```python
from build123d import *

# Parameters (mm, degrees)
SWEEP_THIN1_PROFILE_R   = 30
SWEEP_THIN1_PROFILE_R_2 = 29


with BuildPart() as part:
    # Sweep-Thin1: sweep along a curve in space
    with BuildLine() as sweep_thin1_path:
        Line((-30068.540907505, -16257.859563295, 40521.703196056), (-29659.188972505, -16257.859563295, 40521.703196056))
        ThreePointArc((-29599.188972505, -16197.859563295, 40521.703196056), (-29616.762565634, -16240.285970167, 40521.703196056), (-29659.188972505, -16257.859563295, 40521.703196056))
        Line((-29599.188972505, -16197.859563295, 40521.703196056), (-29599.188972505, -16134.686242211, 40521.703196056))
    # Sweep-Thin1 profile (on start of the path) → Sweep-Thin1 (sweep)
    with BuildSketch(Plane(origin=(-30068.540907505, -16257.859563295, 40521.703196056), x_dir=(0, 0, 1), z_dir=(1, 0, 0))):
        Circle(SWEEP_THIN1_PROFILE_R)
        Circle(SWEEP_THIN1_PROFILE_R_2, mode=Mode.SUBTRACT)
    sweep(path=sweep_thin1_path.line)


solid = part.part
```
Check sheet for the modelled part. Datum: model origin and axes. Units: mm. A direction names the side the tool comes from. Give positions to 0.01 mm unless a question says otherwise; leave off trailing zeros. Write each loop counter-clockwise with the first axis right and the second up, starting at its lowest first coordinate (ties: lowest second). Pieces come first, ordered by that corner, then holes.
Item 1: Cross-section at A-A (z = 40515.5). Enter the section's corners in (x, y), and give its area (3 significant figures).
Item 2: Access from +Z, -Z, +X, -X, +Y, -Y to the whole of each face (thin tool, end or side, straight path). Record for faces 4 (the face through (-29861, -16232.13, 40535.08)), 5 (the face through (-30068.541, -16274, 40497)), 6 (the face through (-29610.679, -16165.831, 40549.416)).
Item 3: Scan lines: L1, parallel to Y at x = -29768.5, z = 40521.5; L2, parallel to Y at x = -29986, z = 40523; L3, parallel to X at y = -16221, z = 40516. Record each from-to range of solid material in increasing order.
Item 4: Cross-section at B-B (y = -16167). Enter the section's corners in (x, z).
Item 5: Draft check along Z on faces 1 (the face through (-29590.478, -16165.831, 40549.364)), 2 (the face through (-29860.999, -16246.369, 40549.416)), 3 (the face through (-29583, -16134.686, 40497)). Enter one of: released by +Z, released by -Z, zero draft, split by the parting line, or undercut.
Item 6: Cross-section at C-C (x = -29787). Enter the section's corners in (y, z).
Item 7: Gauge pin test, flat ends, axial feed: pin 1 (4 mm diameter, centred on y = -16246.5, z = 40528.5, fed in from -X); pin 2 (6 mm diameter, centred on y = -16210, z = 40516, fed in from +X); pin 3 (1.5 mm diameter, centred on x = -29848.5, z = 40510.5, fed in from -Y). Record the tip position at first contact, or that the pin passes through.
Report:
1. outline: (-30068.54, -16287.21) - (-29659.19, -16287.21) arc R89.35 ccw to (-29569.84, -16197.86) - (-29569.84, -16134.69) - (-29570.86, -16134.69) - (-29570.86, -16197.86) arc R88.33 cw to (-29659.19, -16286.19) - (-30068.54, -16286.19) - close; (-30068.54, -16229.53) - (-29659.19, -16229.53) arc R31.67 ccw to (-29627.52, -16197.86) - (-29627.52, -16134.69) - (-29628.54, -16134.69) - (-29628.54, -16197.86) arc R30.65 cw to (-29659.19, -16228.51) - (-30068.54, -16228.51) - close
1. area: 1,160 mm2
2. face 4: -X
2. face 5: +Z, -Z, -X, +Y, -Y
2. face 6: +Y
3. L1: y = -16287.86 to -16286.86, -16228.86 to -16227.86
3. L2: y = -16287.83 to -16286.83, -16228.89 to -16227.89
3. L3: x = -29639.25 to -29637.72, -29573.84 to -29572.78
4. outline: circle Ø60 at (-29599.19, 40521.7); hole circle Ø58 at (-29599.19, 40521.7)
5. face 1: undercut
5. face 2: split by the parting line
5. face 3: zero draft
6. outline: circle Ø60 at (-16257.86, 40521.7); hole circle Ø58 at (-16257.86, 40521.7)
7. pin 1: stops at x = -29587.12
7. pin 2: stops at x = -29569.96
7. pin 3: stops at y = -16285.98
